Geometry: see drawing. Coordinates: mm, zero at the bounding-box minimum. Coordinates: 2 decimals unless noted, no trailing zeros. Write each loop counter-clockwise with the first axis right and the second up, starting at its lowest first coordinate (ties: lowest second). Pieces come first, ordered by that corner, then holes. Notation, with made-up numbers: (50, 41) -> (55, 41) arc R32 cw to (55, 67) -> close; hole circle Ø7 at (1, 56.25). An arc over 180 degrees is marked (long way). Use one line per item in the form item = value. Start each with the question number.
(1) First-contact query: pin 1 (1.8 mm diameter, centred on x = 40, y = 75, fed in from +Z). Flat tip, straight axial feed; report the tip coordinate or a pass-through.
(2) Cut plane B-B on y = 5. Return the cut outline in (x, z), plus the area to 3 significant figures.
(3) Cut plane A-A on x = 95. Return the cut outline in (y, z), plus the area to 3 significant figures.
(4) Ray query, line 1 along X through (y, z) = (77, 1.3); line 2 along Y through (x, z) = (5, 2.25); line 3 along Y through (x, z) = (24.8, 1.65). Return the intervals inside material, ascending.
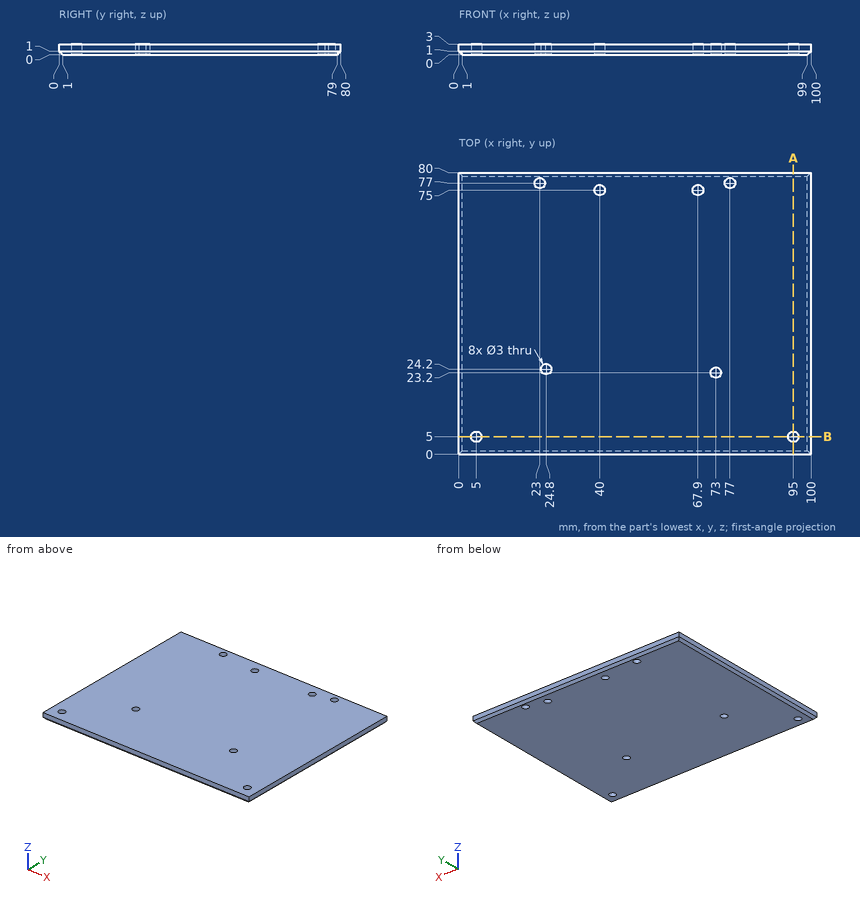
Values:
q1.pin_1 = through
q2.outline = (0, 1) -> (1, 0) -> (3.5, 0) -> (3.5, 3) -> (0, 3) -> close; (6.5, 0) -> (93.5, 0) -> (93.5, 3) -> (6.5, 3) -> close; (96.5, 0) -> (99, 0) -> (100, 1) -> (100, 3) -> (96.5, 3) -> close
q2.area = 281 mm2
q3.outline = (0, 1) -> (1, 0) -> (3.5, 0) -> (3.5, 3) -> (0, 3) -> close; (6.5, 0) -> (79, 0) -> (80, 1) -> (80, 3) -> (6.5, 3) -> close
q3.area = 230 mm2
q4.line_1 = 0 to 21.5, 24.5 to 75.5, 78.5 to 100
q4.line_2 = 0 to 3.5, 6.5 to 80
q4.line_3 = 0 to 22.7, 25.7 to 80
